from build123d import *

# Parameters (mm, degrees)
BOSS_EXTRUDE1_DEPTH   = 4.7625
F_4_CLEARANCE_HOLE1_D = 3.2639
SKETCH10_R            = 2.025
CUT_EXTRUDE1_DEPTH    = 10


with BuildPart() as part:
    # Sketch1 → Boss-Extrude1 (new body)
    with BuildSketch(Plane(origin=(0, 0, 0), x_dir=(0, 0, -1), z_dir=(1, 0, 0))):
        with BuildLine():
            Line((0, 0), (40, 0))
            Line((40, 0), (40, 57.9))
            ThreePointArc((40, 57.9), (37.949747468, 62.849747468), (33, 64.9))
            Line((33, 64.9), (7, 64.9))
            ThreePointArc((7, 64.9), (2.050252532, 62.849747468), (0, 57.9))
            Line((0, 57.9), (0, 0))
        make_face()
    extrude(amount=BOSS_EXTRUDE1_DEPTH)

    # #4 Clearance Hole1 (through all)
    with Locations(Plane(origin=(4.7625, 0, 0), x_dir=(0, 0, -1), z_dir=(1, 0, 0))):
        with Locations((7.5, 5), (20, 5), (32.5, 5)):
            Hole(F_4_CLEARANCE_HOLE1_D / 2)

    # Sketch10 → Cut-Extrude1 (cut)
    with BuildSketch(Plane(origin=(4.7625, 0, 0), x_dir=(0, 0, -1), z_dir=(1, 0, 0))):
        with Locations((20, 57.9)):
            Circle(SKETCH10_R)
    extrude(amount=-CUT_EXTRUDE1_DEPTH, mode=Mode.SUBTRACT)


solid = part.part
Work out the finished part from the listing and answer in its coordinate system (mm). Give positions to 0.01 mm unless a question says otherwise; leave off trailing zeros. Order: outer loops, then holes, each group sorted by start corner. A loop starts at its lowest first (then second) coordinate and runs counter-clockwise, first axis right, second up. Notation, with made-up numbers: (2.5, 23) -> (7.5, 23) arc R26 cw to (7.5, 44) -> close; hole circle Ø9 at (10, 54.25). An arc over 180 degrees is marked (long way). One line per item, written item: value.
Item 1: Determine the mould class of faces 1 (the cylindrical face through (2.3, 62.8, -38)), 2 (the cylindrical face through (2.348, 5.49, -30.943)), 3 (the flat face through (0, 33, -20)) for opening direction Z: released by +Z, released by -Z, zero draft, split by the parting line, or undercut.
Answer sheet:
face 1: released by -Z
face 2: undercut
face 3: zero draft
Item 2: Find section C-C, the plane z = -20. Give the vertices of the cut face in (x, y) (1 decimal).
Answer sheet:
outline: (0, 0) -> (4.8, 0) -> (4.8, 3.4) -> (0, 3.4) -> close; (0, 6.6) -> (4.8, 6.6) -> (4.8, 55.9) -> (0, 55.9) -> close; (0, 59.9) -> (4.8, 59.9) -> (4.8, 64.9) -> (0, 64.9) -> close
Item 3: Straight lines are drawn through the part: probe 1 along Y at (x, z) = (1.8, -20) (3 decimals); probe 2 along Y at (x, z) = (3.35, -32.5); probe 3 along Y at (x, z) = (1.6, -33.5). For each, find the intervals that lie inside material, in ascending order.
Answer sheet:
probe 1: 0 to 3.368, 6.632 to 55.875, 59.925 to 64.9
probe 2: 0 to 3.37, 6.63 to 64.9
probe 3: 0 to 3.71, 6.29 to 64.88
Item 4: Find section B-B, the plane x = 4.1. Give the vertices of the cut face in (y, z) (3 decimals).
Answer sheet:
outline: (0, -40) -> (57.9, -40) arc R7 ccw to (64.9, -33) -> (64.9, -7) arc R7 ccw to (57.9, 0) -> (0, 0) -> close; hole circle Ø3.264 at (5, -32.5); hole circle Ø3.264 at (5, -20); hole circle Ø3.264 at (5, -7.5); hole circle Ø4.05 at (57.9, -20)
Item 5: Find section A-A, the plane y = 5. Give the vertices of the cut face in (x, z).
Answer sheet:
outline: (0, -40) -> (4.76, -40) -> (4.76, -34.13) -> (0, -34.13) -> close; (0, -30.87) -> (4.76, -30.87) -> (4.76, -21.63) -> (0, -21.63) -> close; (0, -18.37) -> (4.76, -18.37) -> (4.76, -9.13) -> (0, -9.13) -> close; (0, -5.87) -> (4.76, -5.87) -> (4.76, 0) -> (0, 0) -> close
